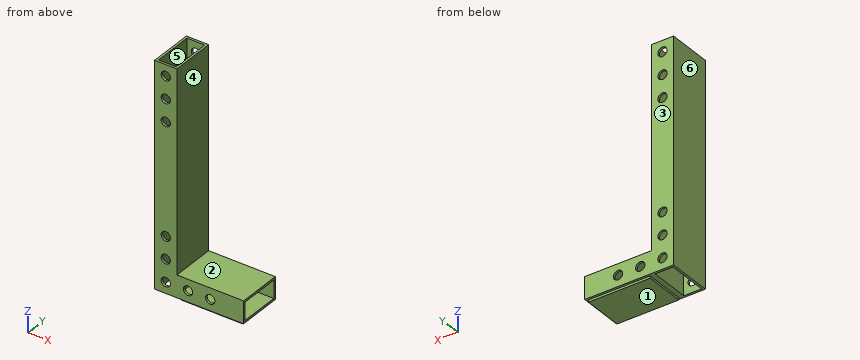
Autodesk Inventor part; units mm, degrees
ref_plane "YZ Plane" through (0, 0, 0) normal (1, 0, 0) x (0, 1, 0)
ref_plane "XZ Plane" through (0, 0, 0) normal (0, 1, 0) x (-1, 0, 0)
ref_plane "XY Plane" through (0, 0, 0) normal (0, 0, 1) x (1, 0, 0)
sketch "Sketch15" plane through (0, 0, 0) normal (1, 0, 0) x (0, 1, 0)
  line L0 (0, 0) -> (50.8, 0)
  line L1 (50.8, 0) -> (50.8, 25.4)
  line L2 (50.8, 25.4) -> (0, 25.4)
  line L3 (0, 25.4) -> (0, 0)
  line L4 (48.26, 22.86) -> (2.54, 22.86)
  line L5 (2.54, 22.86) -> (2.54, 2.54)
  line L6 (2.54, 2.54) -> (48.26, 2.54)
  line L7 (48.26, 2.54) -> (48.26, 22.86)
  dimension "d46" = 25.4
  dimension "d47" = 50.8
  dimension "d48" = 2.54
  dimension "d49" = 2.54
  dimension "d50" = 2.54
  dimension "d51" = 2.54
extrude "Extrusion12" add sketch "Sketch15" along normal blind 76.2
sketch "Sketch17" plane through (0, 0, 0) normal (0, 0, -1) x (-1, 0, 0)
  line L0 (0, 2.54) -> (-76.2, 2.54)
  line L1 (0, 48.26) -> (-76.2, 48.26)
  line L2 (-73.617, 2.54) -> (-3.1161, 2.54)
  line L3 (-3.1161, 2.54) -> (-3.1161, 48.26)
  line L4 (-3.1161, 48.26) -> (-73.617, 48.26)
  line L5 (-73.617, 48.26) -> (-73.617, 2.54)
  point P0 (0, 0)
extrude "Extrusion14" add sketch "Sketch17" along normal blind 2.54
sketch "Sketch20" plane through (0, 0, 0) normal (0, 0, -1) x (-1, 0, 0)
  line L0 (0, 0) -> (25.4, 0)
  line L1 (25.4, 0) -> (0, 0)
  line L2 (0, 0) -> (0, 50.8)
  line L3 (0, 50.8) -> (25.4, 50.8)
  line L4 (25.4, 50.8) -> (25.4, 0)
  line L5 (22.86, 48.26) -> (2.54, 48.26)
  line L6 (2.54, 48.26) -> (2.54, 2.54)
  line L7 (2.54, 2.54) -> (22.86, 2.54)
  line L8 (22.86, 2.54) -> (22.86, 48.26)
  line L9 (0, 0) -> (0, 50.8)
  dimension "d71" = 25.4
  dimension "d72" = 50.8
  dimension "d73" = 2.54
  dimension "d74" = 2.54
  dimension "d75" = 2.54
  dimension "d76" = 2.54
  dimension "d78" = 0
extrude "Extrusion16" add sketch "Sketch20" against normal blind 254
sketch "Sketch21" plane through (76.2, 0, 0) normal (0, -1, 0) x (1, 0, 0)
  circle A0 centre (-38.1, 12.7) radius 5.2917
  circle A1 centre (-63.5, 12.7) radius 5.2917
  circle A2 centre (-88.9, 12.7) radius 5.2917
  circle A3 centre (-88.9, 38.1) radius 5.2917
  circle A4 centre (-88.9, 63.5) radius 5.2917
  line L0 (-76.2, 25.4) -> (0, 25.4)
  line L1 (-101.6, 0) -> (-101.6, 254)
  line L2 (-76.2, 25.4) -> (-76.2, 254)
  point P0 (-76.2, 0)
  dimension "d81" = 12.7
  dimension "d82" = 12.7
  dimension "d83" = 12.7
  dimension "d84" = 25.4
  dimension "d85" = 12.7
  dimension "d86" = 10.5833
  dimension "d87" = 10.5833
  dimension "d88" = 10.5833
  dimension "d89" = 25.4
  dimension "d90" = 25.4
  dimension "d91" = 25.4
  dimension "d92" = 10.5833
  dimension "d93" = 10.5833
  dimension "d94" = 12.7
  dimension "d95" = 12.7
extrude "Extrusion17" cut sketch "Sketch21" against normal blind 76.2
sketch "Sketch22" plane through (76.2, 50.8, 25.4) normal (0, 1, 0) x (1, 0, 0)
  circle A0 centre (-88.9, -215.9) radius 5.2917
  circle A1 centre (-88.9, -190.5) radius 5.2917
  circle A2 centre (-88.9, -165.1) radius 5.2917
  line L0 (-76.2, 0) -> (-76.2, -228.6)
  line L1 (-76.2, -228.6) -> (-101.6, -228.6)
  point P0 (-76.2, 25.4)
  dimension "d98" = 25.4
  dimension "d99" = 25.4
  dimension "d100" = 12.7
  dimension "d101" = 12.7
  dimension "d102" = 12.7
  dimension "d103" = 10.5833
  dimension "d104" = 10.5833
  dimension "d105" = 10.5833
  dimension "d108" = 12.7
extrude "Extrusion18" cut sketch "Sketch22" against normal blind 76.2
equation "\"d49\" = d48"
equation "\"d50\" = d48"
equation "\"d51\" = d48"
equation "\"d73\" = d77"
equation "\"d74\" = d77"
equation "\"d75\" = d77"
equation "\"d76\" = d77"
equation "\"d87\" = d86"
equation "\"d88\" = d86"
equation "\"d92\" = d86"
equation "\"d93\" = d86"
equation "\"d101\" = d100"
equation "\"d102\" = d100"
equation "\"d104\" = d103"
equation "\"d105\" = d103"
properties part number "left arm"
Here's how the part is built. I have some questions about the finished solid (model axes, mm). Face numbers are marked on the shaded views. A direction names the side the tool comes from. Round coordinates to 2 decimals unless told otherwise and drop trailing zeros. Write each loop counter-clockwise with the first axis right and the second up, starting at its lowest first coordinate (ties: lowest second). Pieces come first, ordered by that corner, then holes.
1. Suppose I cut it at A-A (y = 29.5). List the corners of the cut face in (x, z) for me.
2. Suppose I cut it at B-B (z = 215.9). List the corners of the cut face in (x, y) for me, and give its area (3 significant figures).
3. Suppose I cut it at D-D (z = 109). List the corners of the cut face in (x, y) for me, and give its area (3 significant figures).
4. Suppose I cut it at C-C (x = 12.7). List the corners of the cut face in (y, z) for me, and give its area (3 significant figures).
5. I need wall thicknesses on L1, parallel to Y at x = -3, z = 170; L2, parallel to X at y = 28.5, z = 125.5; L3, parallel to Z at x = 60.5, y = 7.5. Which ranges of each line are inside material? Lowest first, please.
6. Will these pins go through, and if not, where does the flat tip stop? pin 1 Ø22.5 at (x, z) = (-12, 66) entering from +Y; pin 2 Ø13.5 at (y, z) = (33, 83.5) entering from +X; pin 3 Ø10 at (x, y) = (52, 5.5) entering from +Z; pin 4 Ø0.8 at (x, z) = (28.5, -1.5) entering from -Y.
7. If we mould it in two halves opening along X, with no side actions, what happens to the marked faces 3, 4, 5 and 6? For each: released by +X, released by -X, zero draft, split by the parting line, or undercut.
8. For the marked faces 1 and 2, which set-ups out of +Z, -Z, +X, -X, +Y, -Y let a thin tool reach every point of the face, with its end or its side?
Answer sheet:
1. outline: (-25.4, 0) - (-22.86, 0) - (-22.86, 254) - (-25.4, 254) - close; (-2.54, 0) - (3.12, 0) - (3.12, -2.54) - (73.62, -2.54) - (73.62, 0) - (76.2, 0) - (76.2, 2.54) - (0, 2.54) - (0, 22.86) - (76.2, 22.86) - (76.2, 25.4) - (0, 25.4) - (0, 254) - (-2.54, 254) - close
2. outline: (-25.4, 0) - (-17.99, 0) - (-17.99, 2.54) - (-22.86, 2.54) - (-22.86, 48.26) - (-17.99, 48.26) - (-17.99, 50.8) - (-25.4, 50.8) - close; (-7.41, 0) - (0, 0) - (0, 50.8) - (-7.41, 50.8) - (-7.41, 48.26) - (-2.54, 48.26) - (-2.54, 2.54) - (-7.41, 2.54) - close
2. area: 308 mm2
3. outline: (-25.4, 0) - (0, 0) - (0, 50.8) - (-25.4, 50.8) - close; hole (-22.86, 2.54) - (-2.54, 2.54) - (-2.54, 48.26) - (-22.86, 48.26) - close
3. area: 361 mm2
4. outline: (0, 0) - (2.54, 0) - (2.54, -2.54) - (48.26, -2.54) - (48.26, 0) - (50.8, 0) - (50.8, 7.41) - (48.26, 7.41) - (48.26, 2.54) - (2.54, 2.54) - (2.54, 7.41) - (0, 7.41) - close; (0, 17.99) - (2.54, 17.99) - (2.54, 22.86) - (48.26, 22.86) - (48.26, 17.99) - (50.8, 17.99) - (50.8, 25.4) - (0, 25.4) - close
4. area: 424 mm2
5. L1: y = 0 to 2.54, 48.26 to 50.8
5. L2: x = -25.4 to -22.86, -2.54 to 0
5. L3: z = -2.54 to 2.54, 22.86 to 25.4
6. pin 1: stops at y = 50.8
6. pin 2: stops at x = 0
6. pin 3: stops at z = 25.4
6. pin 4: stops at y = 2.54
7. face 3: zero draft
7. face 4: released by +X
7. face 5: undercut
7. face 6: released by -X
8. face 1: -Z, +X, -X, +Y, -Y
8. face 2: +Z, +X, +Y, -Y
